Check sheet for the drawn part. Datum: minimum x, y, z corner. Units: mm. Give positions to 0.01 mm unless a question says otherwise; leave off trailing zeros. Loops run counter-clockwise (first coordinate to the right, second up) from the corner with the lowest first, then second, coordinate; pieces in that order, holes last. Notation, with made-up numbers: M 16,-32 L 46,-32 A6 cw 46,-24 Z; hole C 63.5,-11 d5. An arc over 180 degrees is marked long. Write each question's results on one line, items separated by ' | '. Start each with the question number.
1. Sectioned sample at C-C on z = 3.5. Record the cut outline in (x, y).
2. Sectioned sample at D-D on z = 15.5. Record the cut outline in (x, y), and give its area (3 significant figures).
3. Draft check along Y on the marked faces 1, 2 and 3. Enter one of: pulls with the +Y half, pulls with the -Y half, needs draft (parallel to the pull), parting line crosses it, or undercut.
4. Material ranges on line 1 along Y through (x, z) = (10, 12.5); line 2 along Y through (x, z) = (9.5, 11.75); line 3 along X through (y, z) = (12, 10), recorded low to high.
5. Sectioned sample at A-A on x = 10. Record the cut outline in (y, z), and give its area (3 significant figures).
6. Go/stop test with flat-tipped pins: pin 1 (1.5 mm diameter, centred on x = 12, z = 3.5, fed in from -Y); pin 2 (5 mm diameter, centred on y = 12, z = 12, fed in from +X); pin 3 (10 mm diameter, centred on y = 4.5, z = 7, fed in from -X); pin 4 (2.5 mm diameter, centred on x = 10, y = 10, fed in from -Z). Record where each tip stops, or that it passes through.
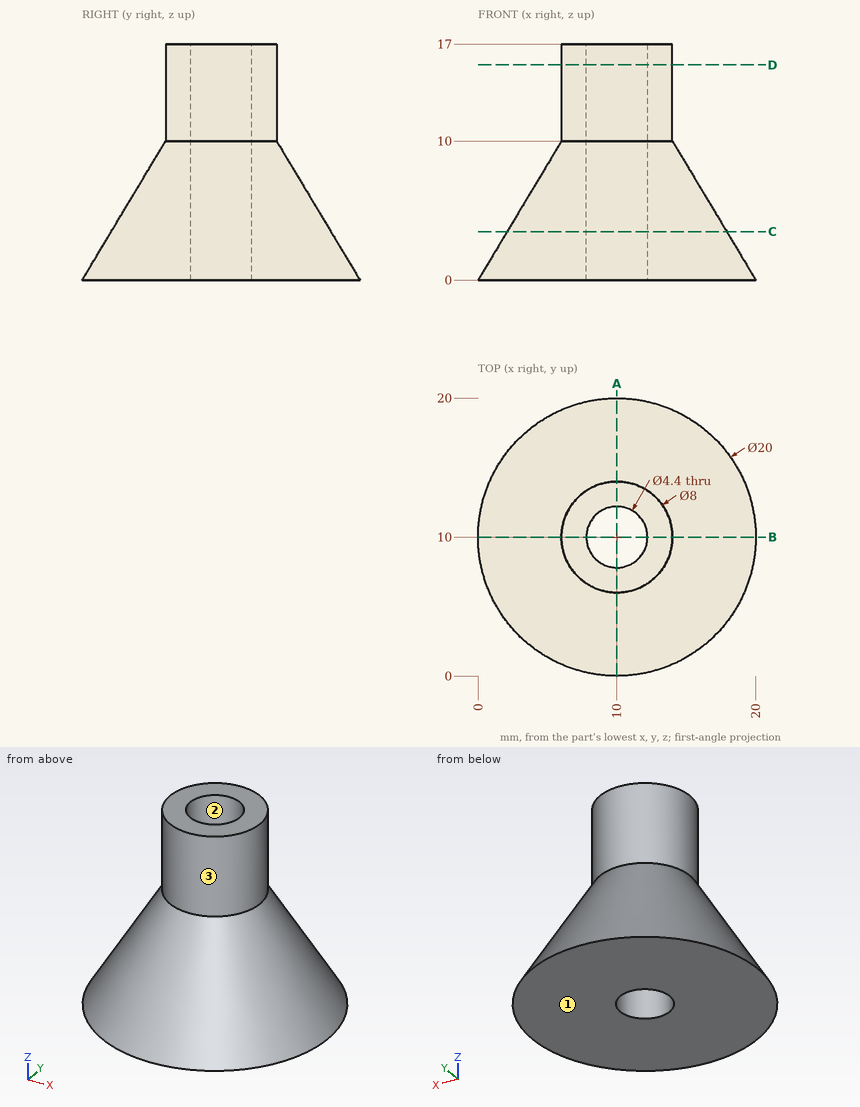
Output values:
1) outline: C 10,10 d15.8; hole C 10,10 d4.4
2) outline: C 10,10 d8; hole C 10,10 d4.4 | area: 35.1 mm2
3) face 1: needs draft | face 2: undercut | face 3: parting line crosses it
4) line 1: 6 to 7.8, 12.2 to 14 | line 2: 6.03 to 7.86, 12.14 to 13.97 | line 3: 6.54 to 9.08, 10.92 to 13.46
5) outline: M 0,0 L 7.8,0 L 7.8,17 L 6,17 L 6,10 Z; M 12.2,0 L 20,0 L 14,10 L 14,17 L 12.2,17 Z | area: 121 mm2
6) pin 1: y = 1.86 | pin 2: x = 14.05 | pin 3: x = 2.16 | pin 4: through
